from build123d import *

# Parameters (mm, degrees)
SKETCH1_R           = 39.6875
BOSS_EXTRUDE1_DEPTH = 12.7
SKETCH2_R           = 37.6555
BOSS_EXTRUDE2_DEPTH = 877.2906
SKETCH3_R           = 28.575
BOSS_EXTRUDE3_DEPTH = 25.7048
SKETCH4_R           = 12.7
BOSS_EXTRUDE4_DEPTH = 19.7358
CHAMFER1_SIZE       = 1


with BuildPart() as part:
    # Sketch1 → Boss-Extrude1 (new body)
    with BuildSketch(Plane.XY):
        Circle(SKETCH1_R)
    extrude(amount=BOSS_EXTRUDE1_DEPTH)

    # Sketch2 → Boss-Extrude2 (add)
    with BuildSketch(Plane.XY.offset(12.7)):
        Circle(SKETCH2_R)
    extrude(amount=BOSS_EXTRUDE2_DEPTH)

    # Sketch3 → Boss-Extrude3 (add)
    with BuildSketch(Plane.XY.offset(889.9906)):
        Circle(SKETCH3_R)
    extrude(amount=BOSS_EXTRUDE3_DEPTH)

    # Sketch4 → Boss-Extrude4 (add)
    with BuildSketch(Plane.XY.offset(915.6954)):
        with Locations(Location((0, 0, 0), (0, 0, 180))):
            Circle(SKETCH4_R)
    extrude(amount=BOSS_EXTRUDE4_DEPTH)

    # Chamfer1
    chamfer1_edges = [part.edges().sort_by_distance(p)[0] for p in [
        (-28.575, 0, 915.6954),
        (12.7, 0, 935.4312),
        (-39.6875, 0, 0),
        (-39.6875, 0, 12.7),
        (-37.6555, 0, 889.9906),
    ]]
    chamfer(chamfer1_edges, length=CHAMFER1_SIZE)


solid = part.part
Geometry check sheet. Reference: the model listing, model coordinates, mm. A direction names the side the tool comes from. Round coordinates to 2 decimals unless told otherwise and drop trailing zeros. Loops run counter-clockwise (first coordinate to the right, second up) from the corner with the lowest first, then second, coordinate; pieces in that order, holes last.
Item 1: Gauge pin test, flat ends, axial feed: pin 1 (2 mm diameter, centred on y = -20.5, z = 236, fed in from +X); pin 2 (3 mm diameter, centred on x = -25, z = 633.5, fed in from -Y); pin 3 (6 mm diameter, centred on y = 5, z = 249, fed in from -X). Record the tip position at first contact, or that the pin passes through.
Item 2: Access from +Z, -Z, +X, -X, +Y, -Y to the whole of each face (thin tool, end or side, straight path). Record for faces 1 (the flat face through (12, -6, 915.695)), 2 (the flat face through (0, 0, 935.431)).
Item 3: Cross-section at C-C on z = 412. Record the boundary of the cut face in (x, y), then the cut area to 3 significant figures.
Item 4: Thickness scan on line 1 (Y direction, x = 2.5, z = 498.5); line 2 (Z direction, x = -8, y = 35.5); line 3 (Z direction, x = -2, y = -13). Record the ranges inside material, lowest first.
Item 5: Cross-section at A-A on y = 0. Record the boundary of the cut face in (x, z) (1 decimal).
Answer sheet:
1. pin 1: stops at x = 32.21
1. pin 2: stops at y = -29.42
1. pin 3: stops at x = -37.6
2. face 1: +Z
2. face 2: +Z, +X, -X, +Y, -Y
3. outline: circle Ø75.31 at (0, 0)
3. area: 4,450 mm2
4. line 1: y = -37.57 to 37.57
4. line 2: z = 0 to 889.99
4. line 3: z = 0 to 915.7
5. outline: (-39.7, 1) - (-38.7, 0) - (38.7, 0) - (39.7, 1) - (39.7, 11.7) - (38.7, 12.7) - (37.7, 12.7) - (37.7, 889) - (36.7, 890) - (28.6, 890) - (28.6, 914.7) - (27.6, 915.7) - (12.7, 915.7) - (12.7, 934.4) - (11.7, 935.4) - (-11.7, 935.4) - (-12.7, 934.4) - (-12.7, 915.7) - (-27.6, 915.7) - (-28.6, 914.7) - (-28.6, 890) - (-36.7, 890) - (-37.7, 889) - (-37.7, 12.7) - (-38.7, 12.7) - (-39.7, 11.7) - close
